Check sheet for the modelled part. Datum: model origin and axes. Units: mm. Face numbers are marked on the shaded views. A direction names the side the tool comes from. Coordinates: 2 decimals unless noted, no trailing zeros. Loops run counter-clockwise (first coordinate to the right, second up) from the corner with the lowest first, then second, coordinate; pieces in that order, holes last.
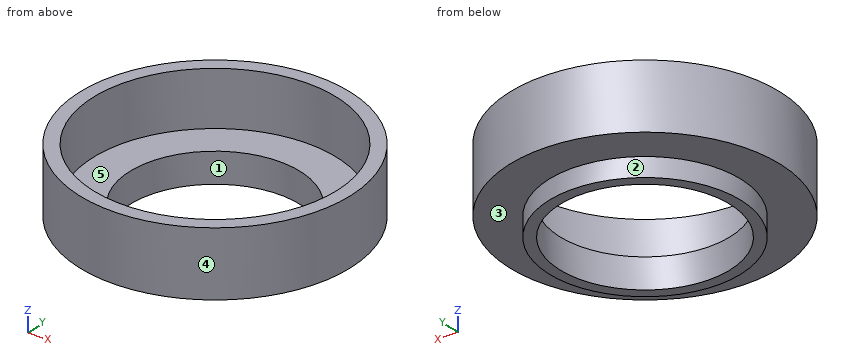
```python
from build123d import *

# Parameters (mm, degrees)
F0_R     = 4.5085
F1_DEPTH = 0.889
F2_R     = 6.35
F4_DEPTH = 3.048
F3_R     = 4.0005
F6_DEPTH = 10.668
F5_R     = 5.715
F7_DEPTH = 2.54


with BuildPart() as f1:
    # F0 (on Top) → F1 (new body)
    with BuildSketch(Plane.XY):
        Circle(F0_R)
    extrude(amount=-F1_DEPTH)

    # F2 (on face) → F4 (join)
    with BuildSketch(Plane.XY):
        Circle(F2_R)
    extrude(amount=F4_DEPTH)

    # F3 (on face) → F6 (cut, symmetric)
    with BuildSketch(Plane.XY):
        Circle(F3_R)
    extrude(amount=F6_DEPTH, both=True, mode=Mode.SUBTRACT)

    # F5 (on face) → F7 (cut)
    with BuildSketch(Plane.XY.offset(3.048)):
        Circle(F5_R)
    extrude(amount=-F7_DEPTH, mode=Mode.SUBTRACT)


solid = f1.part
```
1) Mould release check, pull along X, two halves, no side actions. Record for the marked faces 1, 2 and 3: +X half, -X half, draft (parallel to the pull), parting line (faces both ways), or undercut.
Answer sheet:
face 1: undercut
face 2: parting line
face 3: draft
2) Depth check by flat-ended pin: pin 1 (5 mm diameter, centred on x = -3, y = -3, fed in from +Z); pin 2 (1.5 mm diameter, centred on x = -2.5, z = 0.5, fed in from -Y). Enter the tip coordinate at first touch or a pass-through.
Answer sheet:
pin 1: stops at z = 3.05
pin 2: stops at y = -6.1
3) Scan lines: line 1 (Y direction, x = 0, z = -0.35); line 2 (Y direction, x = 0, z = 1.6) (3 decimals); line 3 (Z direction, x = -3, y = 3.75). Record each from-to range of solid material in increasing order.
Answer sheet:
line 1: y = -4.51 to -4, 4 to 4.51
line 2: y = -6.35 to -5.715, 5.715 to 6.35
line 3: z = 0 to 0.51
4) Section check B-B on y = -3.5. Enter the section's corners in (x, z).
Answer sheet:
outline: (-5.3, 0) - (-2.84, 0) - (-2.84, -0.89) - (-1.94, -0.89) - (-1.94, 0.51) - (-4.52, 0.51) - (-4.52, 3.05) - (-5.3, 3.05) - close; (1.94, -0.89) - (2.84, -0.89) - (2.84, 0) - (5.3, 0) - (5.3, 3.05) - (4.52, 3.05) - (4.52, 0.51) - (1.94, 0.51) - close
5) Section check D-D on y = 4.25. Enter the section's corners in (x, z).
Answer sheet:
outline: (-4.72, 0) - (-1.5, 0) - (-1.5, -0.89) - (1.5, -0.89) - (1.5, 0) - (4.72, 0) - (4.72, 3.05) - (3.82, 3.05) - (3.82, 0.51) - (-3.82, 0.51) - (-3.82, 3.05) - (-4.72, 3.05) - close
6) Section check C-C on z = -0.15. Enter the section's corners in (x, y), plus the area to 3 significant figures.
Answer sheet:
outline: circle Ø9.02 at (0, 0); hole circle Ø8 at (0, 0)
area: 13.6 mm2
7) Set-up check for the marked faces 4 and 5: record each of +Z, -Z, +X, -X, +Y, -Y from which the full face is reachable in a straight line by a thin tool's end or side.
Answer sheet:
face 4: +Z, -Z
face 5: +Z
